```python
from build123d import *

# Parameters (mm, degrees)
SKETCH1_W           = 72.6
SKETCH1_H           = 64
BOSS_EXTRUDE1_DEPTH = 2
SKETCH2_W           = 69.8
SKETCH2_H           = 63.2
BOSS_EXTRUDE2_DEPTH = 1
HOLE1_D             = 3
HOLE1_CBORE_D       = 4.1
HOLE1_CBORE_DEPTH   = 1


with BuildPart() as part:
    # Sketch1 → Boss-Extrude1 (new body)
    with BuildSketch(Plane(origin=(0, 0, 0), x_dir=(1, 0, 0), z_dir=(0, 1, 0))):
        with Locations((36.3, 32)):
            Rectangle(SKETCH1_W, SKETCH1_H)
    extrude(amount=BOSS_EXTRUDE1_DEPTH)

    # Sketch2 → Boss-Extrude2 (add)
    with BuildSketch(Plane(origin=(0, 2, 0), x_dir=(1, 0, 0), z_dir=(0, 1, 0))):
        with Locations((36.3, 31.6)):
            Rectangle(SKETCH2_W, SKETCH2_H)
    extrude(amount=BOSS_EXTRUDE2_DEPTH)

    # Hole1 (through all)
    with Locations(Plane(origin=(0, 3, 0), x_dir=(1, 0, 0), z_dir=(0, 1, 0))):
        with Locations((26.4, 3.5), (46.2, 3.5)):
            CounterBoreHole(HOLE1_D / 2, HOLE1_CBORE_D / 2, HOLE1_CBORE_DEPTH)


solid = part.part
```
Can you work these out from the model? Positions are in its coordinate system, mm. A direction names the side the tool comes from. Coordinates: 2 decimals unless noted, no trailing zeros. Order: outer loops, then holes, each group sorted by start corner. A loop starts at its lowest first (then second) coordinate and runs counter-clockwise, first axis right, second up. Notation, with made-up numbers: (47.25, 76.5) - (67.25, 76.5) arc R17 cw to (67.25, 92.5) - close; hole circle Ø11 at (-19.5, 86). An arc over 180 degrees is marked (long way). Answer in a Markdown table with one row per item.
1. Suppose I cut it at C-C (y = 2.5). Please give me the cut outline in (x, z).
Reply:
| item | result |
|---|---|
| outline | (1.4, -63.2) - (71.2, -63.2) - (71.2, 0) - (1.4, 0) - close; hole circle Ø4.1 at (26.4, -3.5); hole circle Ø4.1 at (46.2, -3.5) |
2. For pin 1 (0.5 mm diameter, centred on x = 23.5, y = 2.5, fed in from -Z), with a flat end and sliding along its axis, tell me the tip position at first contact or that it passes through.
Reply:
| item | result |
|---|---|
| pin 1 | stops at z = -63.2 |
3. Suppose I cut it at A-A (x = 26.4). Please give me the cut outline in (y, z), and give its area (3 significant figures).
Reply:
| item | result |
|---|---|
| outline | (0, -64) - (2, -64) - (2, -63.2) - (3, -63.2) - (3, -5.55) - (2, -5.55) - (2, -5) - (0, -5) - close; (0, -2) - (2, -2) - (2, -1.45) - (3, -1.45) - (3, 0) - (0, 0) - close |
| area | 181 mm^2 |
4. If I drill on line 1 along Z through (x, y) = (26.4, 2.8); line 2 along Z through (x, y) = (26.4, 0.85); line 3 along Z through (x, y) = (24, 2.35), over which ranges is the centre line in solid material (lowest first)?
Reply:
| item | result |
|---|---|
| line 1 | z = -63.2 to -5.55, -1.45 to 0 |
| line 2 | z = -64 to -5, -2 to 0 |
| line 3 | z = -63.2 to 0 |
5. Suppose I cut it at B-B (z = -3.5). Please give me the cut outline in (x, y).
Reply:
| item | result |
|---|---|
| outline | (0, 0) - (24.9, 0) - (24.9, 2) - (24.35, 2) - (24.35, 3) - (1.4, 3) - (1.4, 2) - (0, 2) - close; (27.9, 0) - (44.7, 0) - (44.7, 2) - (44.15, 2) - (44.15, 3) - (28.45, 3) - (28.45, 2) - (27.9, 2) - close; (47.7, 0) - (72.6, 0) - (72.6, 2) - (71.2, 2) - (71.2, 3) - (48.25, 3) - (48.25, 2) - (47.7, 2) - close |
6. If we mould it in two halves opening along X, with no side actions, what happens to faces 1 (the cylindrical face through (28.29, 2.51, -2.71)), 2 (the flat face through (36, 1, -64)), 3 (the flat face through (72.6, 1, -32))? For each: pulls with the +X half, pulls with the -X half, needs draft (parallel to the pull), parting line crosses it, or undercut.
Reply:
| item | result |
|---|---|
| face 1 | undercut |
| face 2 | needs draft |
| face 3 | pulls with the +X half |
7. For faces 4 (the flat face through (36, 3, -32)), 5 (the cylindrical face through (48.155, 2.507, -4.116)), which set-ups out of +Z, -Z, +X, -X, +Y, -Y let a thin tool reach every point of the face, with its end or its side?
Reply:
| item | result |
|---|---|
| face 4 | +Z, -Z, +X, -X, +Y |
| face 5 | +Y |
